from build123d import *

# Parameters (mm, degrees)
BOSS_EXTRUDE1_DEPTH = 20
SKETCH7_R           = 5
CUT_EXTRUDE1_DEPTH  = 20


with BuildPart() as part:
    # Sketch2 → Boss-Extrude1 (new body)
    with BuildSketch(Plane.XY):
        Polygon((0, 0), (30, 0), (30, 10), (15, 20), (0, 20), align=None)
    extrude(amount=-BOSS_EXTRUDE1_DEPTH)

    # Sketch7 → Cut-Extrude1 (cut)
    with BuildSketch(Plane.XY):
        with Locations((15, 10)):
            Circle(SKETCH7_R)
    extrude(amount=-CUT_EXTRUDE1_DEPTH, mode=Mode.SUBTRACT)


solid = part.part
Can you work these out from the model? Positions are in its coordinate system, mm. Give positions to 0.01 mm unless a question says otherwise; leave off trailing zeros. Loops run counter-clockwise (first coordinate to the right, second up) from the corner with the lowest first, then second, coordinate; pieces in that order, holes last. Notation, with made-up numbers: (31.25, 24.25) -> (67.25, 24.25) arc R15 cw to (67.25, 49.25) -> close; hole circle Ø7 at (9.25, -33). An arc over 180 degrees is marked (long way). Write item = value, one per line.
1) Will these pins go through, and if not, where does the flat tip stop? pin 1 (1 mm diameter, centred on x = 21, z = -2.5, fed in from +Y); pin 2 (4 mm diameter, centred on y = 15, z = -15, fed in from +X).
Check result:
pin_1 = 16.33
pin_2 = 25.5
2) Suppose I cut it at A-A on x = 14.25. Write out the boundary of the cut face in (y, z).
Check result:
outline = (0, -20) -> (5.06, -20) -> (5.06, 0) -> (0, 0) -> close; (14.94, -20) -> (20, -20) -> (20, 0) -> (14.94, 0) -> close
3) Suppose I cut it at C-C on z = -11. Write out the boundary of the cut face in (x, y), then the cut area to 3 significant figures.
Check result:
outline = (0, 0) -> (30, 0) -> (30, 10) -> (15, 20) -> (0, 20) -> close; hole circle Ø10 at (15, 10)
area = 446 mm2
4) Thinking about a two-plate mould opening in Y: for faces 1 (the flat face through (15, 0, -10)), 2 (the flat face through (8, 20, -10)), 3 (the cylindrical face through (19.77, 11.5, -9.86)), 4 (the flat face through (11, 6, -20)), which applies, released by +Y, released by -Y, zero draft, split by the parting line, or undercut?
Check result:
face_1 = released by -Y
face_2 = released by +Y
face_3 = undercut
face_4 = zero draft
5) I need wall thicknesses on L1, parallel to Y at x = 15, z = -5.75; L2, parallel to X at y = 5.75, z = -13.75; L3, parallel to X at y = 13.25, z = -4.75 (3 decimals). Which ranges of each line are inside material? Lowest first, please. Write a range as from..to.
Check result:
L1 = 0..5, 15..20
L2 = 0..12.37, 17.63..30
L3 = 0..11.2, 18.8..25.125
6) Suppose I cut it at D-D on y = 18.5. Write out the boundary of the cut face in (x, z), then the cut area to 3 significant figures.
Check result:
outline = (0, -20) -> (17.25, -20) -> (17.25, 0) -> (0, 0) -> close
area = 345 mm2
7) Suppose I cut it at B-B on y = 12.75. Write out the boundary of the cut face in (x, z) (3 decimals), then the cut area to 3 significant figures.
Check result:
outline = (0, -20) -> (10.824, -20) -> (10.824, 0) -> (0, 0) -> close; (19.176, -20) -> (25.875, -20) -> (25.875, 0) -> (19.176, 0) -> close
area = 350 mm2
